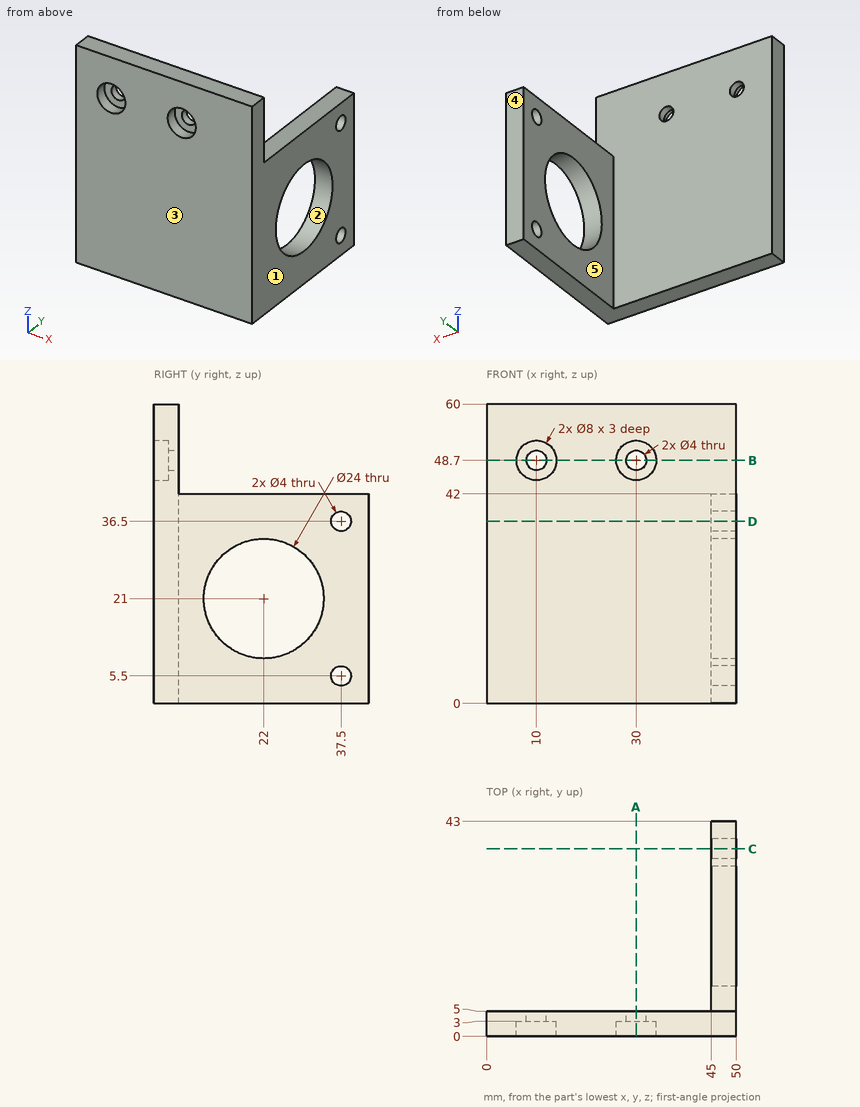
Part print with two shaded views. Sizes in mm from the minimum x, y, z corner. A direction names the side the tool comes from. Round coordinates to 2 decimals unless told otherwise and drop trailing zeros. Order: outer loops, then holes, each group sorted by start corner. A loop starts at its lowest first (then second) coordinate and runs counter-clockwise, first axis right, second up. Notation, with made-up numbers: M 10.5,24.25 L 29.5,24.25 A27 cw 29.5,44.25 Z; hole C 56.5,68 d9. An arc over 180 degrees is marked long. Use CSV: the item, a comma, the result in double quotes.
Item 1: Pin check, flat tips, straight feed: pin 1 (10.5 mm diameter, centred on x = 10, z = 48.7, fed in from +Y); pin 2 (2.5 mm diameter, centred on x = 9.5, z = 47.5, fed in from -Y); pin 3 (5.5 mm diameter, centred on x = 47.5, y = 19.5, fed in from +Z). Stop position of each tip, or through.
Worked answers:
pin 1,"y = 5"
pin 2,"y = 3"
pin 3,"z = 42"
Item 2: Probe probe 1 along X at (y, z) = (4, 48.7); probe 2 along X at (y, z) = (1.1, 48.7); probe 3 along Z at (x, y) = (47.65, 22). List the from-to ranges inside material, lowest first.
Worked answers:
probe 1,"0 to 8, 12 to 28, 32 to 50"
probe 2,"0 to 6, 14 to 26, 34 to 50"
probe 3,"0 to 9, 33 to 42"
Item 3: Saw through at C-C (y = 37.5). List the corners of the cut face in (x, z).
Worked answers:
outline,"M 45,0 L 50,0 L 50,3.5 L 45,3.5 Z; M 45,7.5 L 50,7.5 L 50,34.5 L 45,34.5 Z; M 45,38.5 L 50,38.5 L 50,42 L 45,42 Z"
Item 4: Saw through at A-A (x = 30). List the corners of the cut face in (y, z), plus the area to 3 significant figures.
Worked answers:
outline,"M 0,0 L 5,0 L 5,46.7 L 3,46.7 L 3,44.7 L 0,44.7 Z; M 0,52.7 L 3,52.7 L 3,50.7 L 5,50.7 L 5,60 L 0,60 Z"
area,"268 mm²"
Item 5: Saw through at D-D (z = 36.5). List the corners of the cut face in (x, y).
Worked answers:
outline,"M 0,0 L 50,0 L 50,35.5 L 45,35.5 L 45,5 L 0,5 Z; M 45,39.5 L 50,39.5 L 50,43 L 45,43 Z"
Item 6: Saw through at B-B (z = 48.7). List the corners of the cut face in (x, y).
Worked answers:
outline,"M 0,0 L 6,0 L 6,3 L 8,3 L 8,5 L 0,5 Z; M 12,3 L 14,3 L 14,0 L 26,0 L 26,3 L 28,3 L 28,5 L 12,5 Z; M 32,3 L 34,3 L 34,0 L 50,0 L 50,5 L 32,5 Z"
Item 7: Pull direction Y, two halves, no side cores. Call the marked faces 1, 2 and 3: released by +Y, released by -Y, zero draft, split by the parting line, or undercut.
Worked answers:
face 1,"zero draft"
face 2,"undercut"
face 3,"released by -Y"
Item 8: Which spindle directions (+Z, -Z, +X, -X, +Y, -Y) get a long thin tool onto all of the face, cutting with end or side? Do the marked faces 4 and 5. Say none if no direction does.
Worked answers:
face 4,"+Z, -Z, +X, -X, +Y"
face 5,"+Z, -Z, -X, +Y"
